Autodesk Inventor part; units mm, degrees
ref_plane "YZ Plane" through (0, 0, 0) normal (1, 0, 0) x (0, 1, 0)
ref_plane "XZ Plane" through (0, 0, 0) normal (0, 1, 0) x (-1, 0, 0)
ref_plane "XY Plane" through (0, 0, 0) normal (0, 0, 1) x (1, 0, 0)
sketch "Sketch2" plane through (0, 0, 0) normal (0, 0, 1) x (1, 0, 0)
  arc A0 (20.126, -22.2473) -> (-20.126, -22.2473) centre (0, 0) ccw construction
  arc A1 (-24.3711, -22.2497) -> (-24.3711, 22.2497) centre (0, 0) ccw
  line L0 (32.9543, 32.9543) -> (23.3345, 23.3345) construction
  line L1 (-32.8174, 32.8174) -> (-23.3345, 23.3345) construction
  line L2 (23.3345, 23.3345) -> (-23.3345, -23.3345) construction
  line L3 (23.3345, -23.3345) -> (30.6779, -35.5804) construction
  line L4 (-23.3345, -23.3345) -> (-31.805, -34.2596) construction
  line L5 (-23.3345, 23.3345) -> (23.3345, -23.3345) construction
  line L6 (0, -33) -> (0, 33) construction
  line L7 (32.9543, 0) -> (-32.9543, 0) construction
  circle A2 centre (0, 0) radius 1.5
  circle A3 centre (0, 0) radius 4.5
  line L8 (4.0607, -1.9393) -> (22.2473, -20.126) construction
  line L9 (1.9393, -4.0607) -> (17.8, -19.9213) construction
  arc A4 (0, -30) -> (17.8, -24.1487) centre (0, 0) ccw construction
  line L10 (-1.9393, -4.0607) -> (-17.8, -19.9213) construction
  line L11 (-4.0607, -1.9393) -> (-22.2473, -20.126) construction
  line L12 (23.3345, 23.3345) -> (-23.3345, -23.3345) construction
  arc A5 (-20.126, -22.2473) -> (-17.8, -24.1487) centre (0, 0) ccw construction
  line L13 (17.8, -24.1487) -> (17.8, -19.9213) construction
  line L14 (-17.8, -24.1487) -> (-17.8, -19.9213) construction
  line L15 (17.8, -22.035) -> (-17.8, -22.035) construction
  arc A6 (-17.8, -24.1487) -> (0, -30) centre (0, 0) ccw construction
  line L16 (-17.8, -19.9213) -> (-20.126, -22.2473) construction
  line L17 (17.8, -19.9213) -> (20.126, -22.2473) construction
  arc A7 (17.8, -24.1487) -> (20.126, -22.2473) centre (0, 0) ccw construction
  line L18 (17.8, 19.9213) -> (20.126, 22.2473) construction
  arc A8 (20.126, 22.2473) -> (17.8, 24.1487) centre (0, 0) ccw construction
  arc A9 (-17.8, 24.1487) -> (-20.126, 22.2473) centre (0, 0) ccw construction
  line L19 (-17.8, 19.9213) -> (-20.126, 22.2473) construction
  line L20 (-1.9393, 4.0607) -> (-17.8, 19.9213) construction
  line L21 (1.9393, 4.0607) -> (17.8, 19.9213) construction
  line L22 (17.8, 24.1487) -> (17.8, 19.9213) construction
  arc A10 (17.8, 24.1487) -> (0, 30) centre (0, 0) ccw construction
  arc A11 (0, 30) -> (-17.8, 24.1487) centre (0, 0) ccw construction
  line L23 (-17.8, 24.1487) -> (-17.8, 19.9213) construction
  line L24 (4.0607, 1.9393) -> (22.2473, 20.126) construction
  line L25 (-4.0607, 1.9393) -> (-22.2473, 20.126) construction
  line L26 (-4.0607, 1.9393) -> (-24.3711, 22.2497)
  line L27 (-4.0607, -1.9393) -> (-24.3711, -22.2497)
  arc A12 (-24.3711, 22.2497) -> (-24.3711, -22.2497) centre (0, 0) ccw construction
  line L28 (24.1487, 17.8) -> (19.9213, 17.8)
  line L29 (4.0607, 1.9393) -> (19.9213, 17.8)
  arc A13 (30, 0) -> (24.1487, 17.8) centre (0, 0) ccw
  arc A14 (24.1487, -17.8) -> (30, 0) centre (0, 0) ccw
  line L30 (24.1487, -17.8) -> (19.9213, -17.8)
  line L31 (4.0607, -1.9393) -> (19.9213, -17.8)
  point P0 (0, -22.035)
  point P1 (22.035, 17.8)
  point P2 (22.035, -17.8)
  dimension "d32" = 60
  dimension "d33" = 3
  dimension "d34" = 3
  dimension "d35" = 3
  dimension "d36" = 1.5
  dimension "d37" = 3
  dimension "d38" = 35.6
  dimension "d43" = 45
  dimension "d47" = 90
extrude "Extrusion2" add sketch "Sketch2" along normal blind 60 contours L27 A3 L31 L30 A14 A13 L28 L29 L26 A1 | A3 | A2
fillet "Fillet2" radius 2 10 edges at (-24.3711, 22.2497, 30) (-24.3711, -22.2497, 30) (-4.0607, -1.9393, 30) (-4.0607, 1.9393, 30) (4.0607, -1.9393, 30) (4.0607, 1.9393, 30) (19.9213, -17.8, 30) (24.1487, -17.8, 30) (19.9213, 17.8, 30) (24.1487, 17.8, 30)
properties part number "Feeder Rotator" material "ABS Plastic"
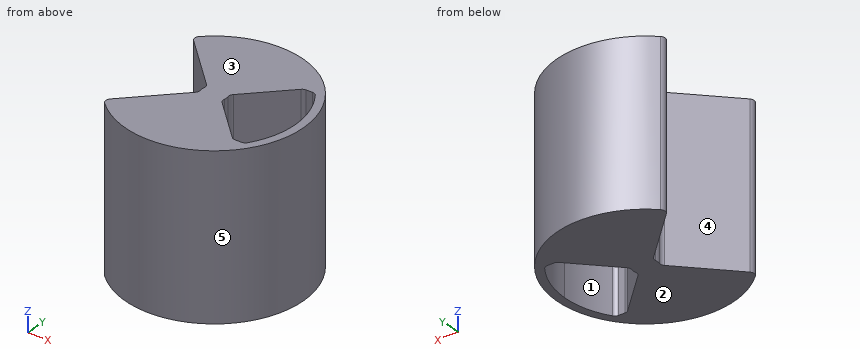
Here's how the part is built. I have some questions about the finished solid (model axes, mm). Face numbers are marked on the shaded views. A direction names the side the tool comes from. Round coordinates to 2 decimals unless told otherwise and drop trailing zeros. Order: outer loops, then holes, each group sorted by start corner. A loop starts at its lowest first (then second) coordinate and runs counter-clockwise, first axis right, second up. Notation, with made-up numbers: (56.25, -36.75) -> (86.25, -36.75) arc R20 ccw to (86.25, -30.75) -> close; hole circle Ø4 at (24.5, 71.5). An arc over 180 degrees is marked (long way). Use a Markdown table: item, result. Add a question column.
(1) Suppose I cut it at A-A, the plane x = 7. Please give me the cut outline in (y, z).
(2) For the marked faces 1 and 2, which set-ups out of +Z, -Z, +X, -X, +Y, -Y let a thin tool reach every point of the face, with its end or its side?
(3) I need wall thicknesses on line 1 along X through (y, z) = (1, 30); line 2 along Y through (x, z) = (-13, 50.5); line 3 along Y through (x, z) = (25, 11). Which ranges of each line are inside material? Lowest first, please.
(4) Suppose I cut it at C-C, the plane z = 31.5. Please give me the cut outline in (x, y), and give its area (3 significant figures).
(5) Suppose I cut it at B-B, the plane y = 12.5. Please give me the cut outline in (x, z).
(6) If we mould it in two halves opening along Y, with no side actions, what happens to the marked faces 3, 4 and 5? For each: released by +Y, released by -Y, zero draft, split by the parting line, or undercut.
(7) Suppose I cut it at D-D, the plane y = -29. Please give me the cut outline in (x, z), and give its area (3 significant figures).
(8) For pin 1 Ø1 at (y, z) = (18, 15.5) entering from -X; pin 2 Ø1.5 at (y, z) = (24, 41) entering from -X; pin 3 Ø1.9 at (x, z) = (22.5, 36) entering from -Y, each with a flat end and sliding along its axis, tell me the tip position at first contact or that it passes through.
Verdict:
| question | item | result |
|---|---|---|
| 1 | outline | (-32.25, 0) -> (-4.88, 0) -> (-4.88, 60) -> (-32.25, 60) -> close; (4.88, 0) -> (32.25, 0) -> (32.25, 60) -> (4.88, 60) -> close |
| 2 | face 1 | +Z, -Z |
| 2 | face 2 | -Z, +X, -X, +Y, -Y |
| 3 | line 1 | -4.39 to 4.39, 29.98 to 32.98 |
| 3 | line 2 | -30.33 to -10.88, 10.88 to 30.33 |
| 3 | line 3 | -21.54 to -16.58, 16.58 to 21.54 |
| 4 | outline | (-22.98, -20.86) arc R2 ccw to (-22.96, -23.71) arc R33 ccw (long way) to (-22.96, 23.71) arc R2 ccw to (-22.98, 20.86) -> (-4.93, 2.81) arc R2 cw to (-4.39, 0.97) arc R4.5 ccw to (-4.39, -0.97) arc R2 cw to (-4.93, -2.81) -> close; hole (4.39, -0.97) arc R2 ccw to (4.93, -2.81) -> (19.34, -17.21) arc R2 ccw to (20.75, -17.8) -> (23.12, -17.8) arc R2 ccw to (24.77, -16.93) arc R30 ccw to (30, 0) arc R30 ccw to (24.77, 16.93) arc R2 ccw to (23.12, 17.8) -> (20.75, 17.8) arc R2 ccw to (19.34, 17.21) -> (4.93, 2.81) arc R2 ccw to (4.39, 0.97) arc R4.5 cw to start |
| 4 | area | 2,060 mm2 |
| 5 | outline | (-14.62, 0) -> (14.62, 0) -> (14.62, 60) -> (-14.62, 60) -> close; (27.27, 0) -> (30.54, 0) -> (30.54, 60) -> (27.27, 60) -> close |
| 6 | face 3 | zero draft |
| 6 | face 4 | undercut |
| 6 | face 5 | split by the parting line |
| 7 | outline | (-15.75, 0) -> (15.75, 0) -> (15.75, 60) -> (-15.75, 60) -> close |
| 7 | area | 1,890 mm2 |
| 8 | pin 1 | x = -20.62 |
| 8 | pin 2 | x = -23.31 |
| 8 | pin 3 | y = -24.99 |
